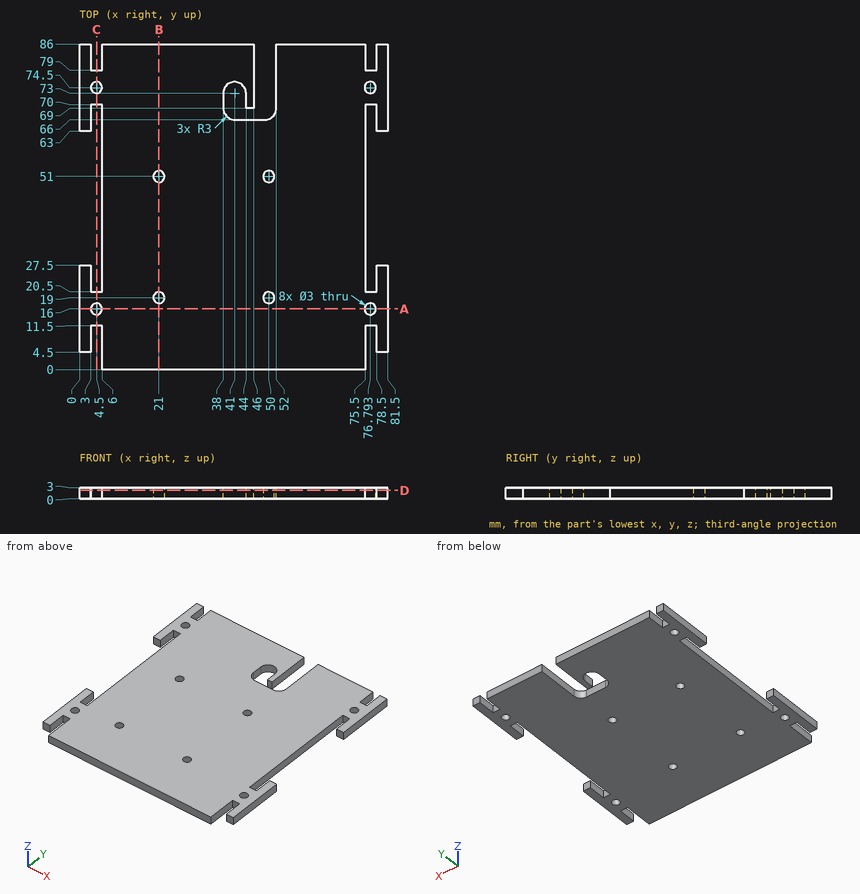
Here's the drawing with two shaded views (mm, measured from the low corner). I have some questions. Give positions to 0.01 mm unless a question says otherwise; leave off trailing zeros. Order: outer loops, then holes, each group sorted by start corner. A loop starts at its lowest first (then second) coordinate and runs counter-clockwise, first axis right, second up. Notation, with made-up numbers: (-26.5, -40) -> (25.5, -40) arc R29 ccw to (25.5, -20) -> close; hole circle Ø8 at (87.25, 49). An arc over 180 degrees is marked (long way). Use a Markdown table: item, result. Add a question column.
Item 1: Imagine slicing it at B-B on x = 21. Please give me the cut outline in (y, z), plus the area to 3 significant figures.
Item 2: Imagine slicing it at C-C on x = 4.5. Please give me the cut outline in (y, z), plus the area to 3 significant figures.
Item 3: Imagine slicing it at A-A on y = 16. Please give me the cut outline in (x, z), plus the area to 4 significant figures.
Item 4: Imagine slicing it at D-D on z = 2.25. Give the number of separate pieces and of enclosed holes in the cut face, plus the area to 3 significant figures.
Item 5: I need wall thicknesses on line 1 (X direction, y = 51, z = 1); line 2 (X direction, y = 19, z = 1.25); line 3 (Y direction, x = 21, z = 2.25). Which ranges of each line are inside material? Lowest first, please.
Item 6: Will this pin go through, and if not, where does the flat tip stop? pin 1 (2.5 mm diameter, centred on x = 4.5, y = 74.5, fed in from -Z).
Data:
| question | item | result |
|---|---|---|
| 1 | outline | (0, 0) -> (17.5, 0) -> (17.5, 3) -> (0, 3) -> close; (20.5, 0) -> (49.5, 0) -> (49.5, 3) -> (20.5, 3) -> close; (52.5, 0) -> (86, 0) -> (86, 3) -> (52.5, 3) -> close |
| 1 | area | 240 mm² |
| 2 | outline | (11.5, 0) -> (14.5, 0) -> (14.5, 3) -> (11.5, 3) -> close; (17.5, 0) -> (20.5, 0) -> (20.5, 3) -> (17.5, 3) -> close; (70, 0) -> (73, 0) -> (73, 3) -> (70, 3) -> close; (76, 0) -> (79, 0) -> (79, 3) -> (76, 3) -> close |
| 2 | area | 36.0 mm² |
| 3 | outline | (0, 0) -> (3, 0) -> (3, 3) -> (0, 3) -> close; (6, 0) -> (75.29, 0) -> (75.29, 3) -> (6, 3) -> close; (78.29, 0) -> (81.5, 0) -> (81.5, 3) -> (78.29, 3) -> close |
| 3 | area | 226.5 mm² |
| 4 | separate pieces | 1 |
| 4 | enclosed holes | 8 |
| 4 | area | 6,130 mm² |
| 5 | line 1 | x = 6 to 19.5, 22.5 to 48.5, 51.5 to 75.5 |
| 5 | line 2 | x = 0 to 19.5, 22.5 to 48.5, 51.5 to 81.5 |
| 5 | line 3 | y = 0 to 17.5, 20.5 to 49.5, 52.5 to 86 |
| 6 | pin 1 | passes through |
